Check sheet for the modelled part. Datum: model origin and axes. Units: mm. A direction names the side the tool comes from. Give positions to 0.01 mm unless a question says otherwise; leave off trailing zeros. Order: outer loops, then holes, each group sorted by start corner. A loop starts at its lowest first (then second) coordinate and runs counter-clockwise, first axis right, second up.
```python
from build123d import *

# Parameters (mm, degrees)
SKETCH1_W           = 70
SKETCH1_H           = 70
BOSS_EXTRUDE1_DEPTH = 2
SKETCH2_W           = 2
SKETCH2_H           = 20
BOSS_EXTRUDE2_DEPTH = 2
SKETCH3_W           = 20
SKETCH3_H           = 2
CUT_EXTRUDE1_DEPTH  = 2
SKETCH4_W           = 10.48
SKETCH4_H           = 5
CUT_EXTRUDE2_DEPTH  = 10


with BuildPart() as part:
    # Sketch1 → Boss-Extrude1 (new body)
    with BuildSketch(Plane.XY):
        Rectangle(SKETCH1_W, SKETCH1_H)
    extrude(amount=-BOSS_EXTRUDE1_DEPTH)

    # Sketch2 → Boss-Extrude2 (add)
    with BuildSketch(Plane.XY):
        with Locations((-36, 15)):
            Rectangle(SKETCH2_W, SKETCH2_H)
        with Locations((-36, -15)):
            Rectangle(SKETCH2_W, SKETCH2_H)
        with Locations((36, -15)):
            Rectangle(SKETCH2_W, SKETCH2_H)
        with Locations((36, 15)):
            Rectangle(SKETCH2_W, SKETCH2_H)
    extrude(amount=-BOSS_EXTRUDE2_DEPTH)

    # Sketch3 → Cut-Extrude1 (cut)
    with BuildSketch(Plane.XY):
        with Locations((-15, 34)):
            Rectangle(SKETCH3_W, SKETCH3_H)
        with Locations((15, 34)):
            Rectangle(SKETCH3_W, SKETCH3_H)
        with Locations((-15, -34)):
            Rectangle(SKETCH3_W, SKETCH3_H)
        with Locations((15, -34)):
            Rectangle(SKETCH3_W, SKETCH3_H)
    extrude(amount=-CUT_EXTRUDE1_DEPTH, mode=Mode.SUBTRACT)

    # Sketch4 → Cut-Extrude2 (cut)
    with BuildSketch(Plane.XY):
        Rectangle(SKETCH4_W, SKETCH4_H)
    extrude(amount=-CUT_EXTRUDE2_DEPTH, mode=Mode.SUBTRACT)


solid = part.part
```
(1) Release check for a two-part mould opening along Y. For faces 5 (the face through (15, -33, -1)), 6 (the face through (-36, -5, -1)), 7 (the face through (-36, 5, -1)), 8 (the face through (-37, 15, -1)) record: released by +Y, released by -Y, zero draft, split by the parting line, or undercut.
Response values:
face 5: released by -Y
face 6: undercut
face 7: undercut
face 8: zero draft
(2) Set-up check for faces 1 (the face through (36, 25, -1)), 2 (the face through (-35, 30, -1)), 3 (the face through (5, 34, -1)), 4 (the face through (36, 5, -1)): record each of +Z, -Z, +X, -X, +Y, -Y from which the full face is reachable in a straight line by a thin tool's end or side.
Response values:
face 1: +Z, -Z, +X, +Y
face 2: +Z, -Z, -X, +Y
face 3: +Z, -Z, +Y
face 4: +Z, -Z, +X
(3) Cross-section at A-A on y = -1. Enter the section's corners in (x, z), then the cut area to 3 significant figures.
Response values:
outline: (-35, -2) - (-5.24, -2) - (-5.24, 0) - (-35, 0) - close; (5.24, -2) - (35, -2) - (35, 0) - (5.24, 0) - close
area: 119 mm2
(4) Material ranges on L1, parallel to X at y = 1.5, z = -1.7; L2, parallel to Y at x = -2.5, z = -1.75; L3, parallel to Y at x = 15.5, z = -1.3, recorded low to high.
Response values:
L1: x = -35 to -5.24, 5.24 to 35
L2: y = -35 to -2.5, 2.5 to 35
L3: y = -33 to 33
(5) Cross-section at B-B on x = 12. Enter the section's corners in (y, z).
Response values:
outline: (-33, -2) - (33, -2) - (33, 0) - (-33, 0) - close
(6) Gauge pin test, flat ends, axial feed: pin 1 Ø0.6 at (y, z) = (1, -1) entering from -X; pin 2 Ø0.6 at (y, z) = (-2, -1) entering from +X; pin 3 Ø1 at (x, z) = (-36, -1) entering from -Y. Record the tip position at first contact, or that the pin passes through.
Response values:
pin 1: stops at x = -35
pin 2: stops at x = 35
pin 3: stops at y = -25
